```python
from build123d import *

# Parameters (mm, degrees)
SKETCH1_W               = 254
SKETCH1_H               = 254
BOSS_EXTRUDE1_DEPTH     = 12.7
CUT_EXTRUDE2_DEPTH      = 181.05357536
CUT_EXTRUDE2_DEPTH_BACK = 181.05357536
SKETCH6_R               = 3.175
CUT_EXTRUDE3_DEPTH      = 181.05357536
CUT_EXTRUDE3_DEPTH_BACK = 181.05357536
SKETCH7_R               = 2.0828


with BuildPart() as part:
    # Sketch1 → Boss-Extrude1 (new body)
    with BuildSketch(Plane(origin=(0, 0, 0), x_dir=(1, 0, 0), z_dir=(0, 1, 0))):
        Rectangle(SKETCH1_W, SKETCH1_H)
    extrude(amount=BOSS_EXTRUDE1_DEPTH)

    # Sketch6 → Cut-Extrude2 (cut, two sides: drawn at the far end of the back side and taken through both)
    with BuildSketch(Plane(origin=(0, 12.7, 0), x_dir=(1, 0, 0), z_dir=(0, 1, 0)).offset(-CUT_EXTRUDE2_DEPTH_BACK)):
        with Locations(Location((0, 63.5, 0), (0, 0, 270))):
            Circle(SKETCH6_R)
        with Locations(Location((44.901280605, 44.901280605, 0), (0, 0, 270))):
            Circle(SKETCH6_R)
        with Locations(Location((63.5, 0, 0), (0, 0, 270))):
            Circle(SKETCH6_R)
        with Locations(Location((44.901280605, -44.901280605, 0), (0, 0, 270))):
            Circle(SKETCH6_R)
        with Locations(Location((0, -63.5, 0), (0, 0, 270))):
            Circle(SKETCH6_R)
        with Locations(Location((-44.901280605, -44.901280605, 0), (0, 0, 270))):
            Circle(SKETCH6_R)
        with Locations(Location((-63.5, 0, 0), (0, 0, 270))):
            Circle(SKETCH6_R)
        with Locations(Location((-44.901280605, 44.901280605, 0), (0, 0, 270))):
            Circle(SKETCH6_R)
    extrude(amount=CUT_EXTRUDE2_DEPTH + CUT_EXTRUDE2_DEPTH_BACK, mode=Mode.SUBTRACT)

    # Sketch7 → Cut-Extrude3 (cut, two sides: drawn at the far end of the back side and taken through both)
    with BuildSketch(Plane(origin=(0, 12.7, 0), x_dir=(1, 0, 0), z_dir=(0, 1, 0)).offset(-CUT_EXTRUDE3_DEPTH_BACK)):
        with Locations(Location((-82.55, 0, 0), (0, 0, 270))):
            Circle(SKETCH7_R)
        with Locations(Location((82.55, 0, 0), (0, 0, 270))):
            Circle(SKETCH7_R)
    extrude(amount=CUT_EXTRUDE3_DEPTH + CUT_EXTRUDE3_DEPTH_BACK, mode=Mode.SUBTRACT)


solid = part.part
```
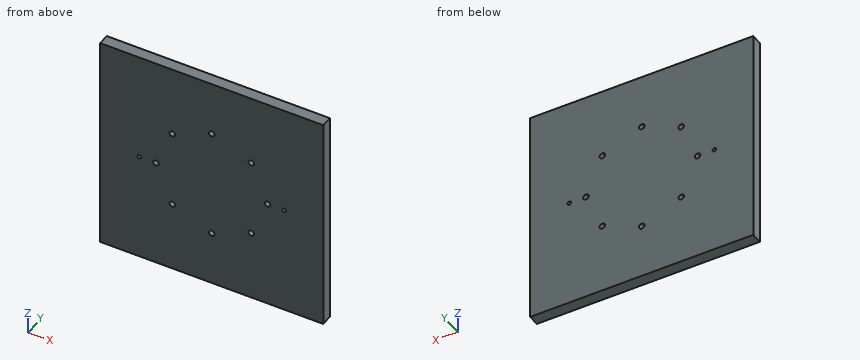
Here's how the part is built. I have some questions about the finished solid (model axes, mm). Round coordinates to 2 decimals unless told otherwise and drop trailing zeros. Order: outer loops, then holes, each group sorted by start corner. A loop starts at its lowest first (then second) coordinate and runs counter-clockwise, first axis right, second up. Notation, with made-up numbers: M 56,48 L 76,48 A10 cw 76,60 Z; hole C 84,-33.5 d2. An arc over 180 degrees is marked long. One line per question, with ' | ' between items.
1) I want a section at B-B, the plane x = 0. Write out the boundary of the cut face in (y, z) (3 decimals), then the cut area to 3 significant figures.
Working result:
outline: M 0,-127 L 12.7,-127 L 12.7,-66.675 L 0,-66.675 Z; M 0,-60.325 L 12.7,-60.325 L 12.7,60.325 L 0,60.325 Z; M 0,66.675 L 12.7,66.675 L 12.7,127 L 0,127 Z | area: 3,060 mm²
2) I need wall thicknesses on line 1 along Z through (x, y) = (0, 3.25) (3 decimals); line 2 along X through (y, z) = (4.75, 0) (3 decimals); line 3 along Z through (x, y) = (64, 6.5). Which ranges of each line are inside material? Lowest first, please.
Working result:
line 1: -127 to -66.675, -60.325 to 60.325, 66.675 to 127 | line 2: -127 to -84.633, -80.467 to -66.675, -60.325 to 60.325, 66.675 to 80.467, 84.633 to 127 | line 3: -127 to -3.14, 3.14 to 127
3) I want a section at A-A, the plane z = -63.5. Write out the boundary of the cut face in (x, y) (3 decimals), then the cut area to 3 significant figures.
Working result:
outline: M -127,0 L -3.175,0 L -3.175,12.7 L -127,12.7 Z; M 3.175,0 L 127,0 L 127,12.7 L 3.175,12.7 Z | area: 3,150 mm²
4) For pin 1 Ø3.5 at (x, z) = (-82.55, 0) entering from +Y, with a flat end and sliding along its axis, tell me the tip position at first contact or that it passes through.
Working result:
pin 1: through
